Verification items for the finished model (mm, model axes). Face numbers are marked on the shaded views. Round coordinates to 2 decimals unless told otherwise and drop trailing zeros. Loops run counter-clockwise (first coordinate to the right, second up) from the corner with the lowest first, then second, coordinate; pieces in that order, holes last. Notation, with made-up numbers: M -15,-21 L 16,-21 A22 ccw 16,4 Z; hole C -18.5,3.25 d7. An arc over 180 degrees is marked long. One line per item, written item: value.
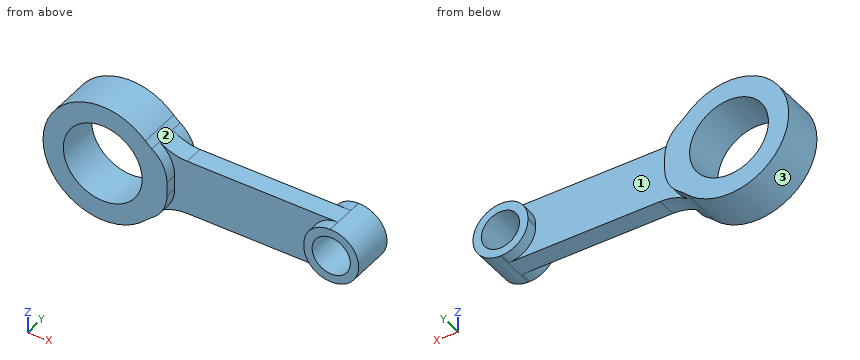
from build123d import *

# Parameters (mm, degrees)
F0_R          = 16.5
F0_R_2        = 8
F1_DEPTH      = 17.9
F2_W          = 57.2901275009
F2_H          = 11.0436469637
F2_H_2        = 10.7600754127
F3_DEPTH      = 25.001
F3_DEPTH_BACK = 25.001
F4_R          = 11
F5_R          = 11
F6_R          = 11
F7_R          = 15


with BuildPart() as f1:
    # F0 (on Front) → F1 (new body)
    with BuildSketch(Plane.XZ):
        with BuildLine():
            Line((32.137329833, -11.4990798469), (95.5545260385, -11.4990798469))
            Line((95.5545260385, -11.4990798469), (95.8454739615, -11.4990798469))
            ThreePointArc((95.8454739615, -11.4990798469), (107.1962842582, 0.2923153343), (95.2608909699, 11.4916136056))
            Line((95.2608909699, 11.4916136056), (32.1446460941, 11.4916136056))
            ThreePointArc((32.1446460941, 11.4916136056), (24.3962738222, 13.0535354211), (17.858136719, 17.495340892))
            ThreePointArc((17.858136719, 17.495340892), (-24.9999998314, 0.0029037072), (17.8540721294, -17.4994888039))
            ThreePointArc((17.8540721294, -17.4994888039), (24.3910991645, -13.0601018267), (32.137329833, -11.4990798469))
        make_face()
        Circle(F0_R, mode=Mode.SUBTRACT)
        with Locations((95.7, 0)):
            Circle(F0_R_2, mode=Mode.SUBTRACT)
    extrude(amount=F1_DEPTH)

    # F2 (on Top) → F3 (cut, two sides)
    with BuildSketch(Plane.XY) as f3_sk:
        with Locations((55.5549362496, 0.6468234818)):
            Rectangle(F2_W, F2_H)
        with Locations((55.5549362496, -18.4050377063)):
            Rectangle(F2_W, F2_H_2)
    extrude(amount=-F3_DEPTH, mode=Mode.SUBTRACT)
    extrude(f3_sk.sketch, amount=F3_DEPTH_BACK, mode=Mode.SUBTRACT)

    # F4
    f4_edges = [f1.edges().sort_by_distance(p)[0] for p in [
        (84.2, -2.4375, -11.49908),
    ]]
    fillet(f4_edges, radius=F4_R)

    # F5
    f5_edges = [f1.edges().sort_by_distance(p)[0] for p in [
        (84.2, -2.4375, 11.491614),
    ]]
    fillet(f5_edges, radius=F5_R)

    # F6
    f6_edges = [f1.edges().sort_by_distance(p)[0] for p in [
        (84.2, -15.4625, -11.49908),
        (84.2, -15.4625, 11.491614),
    ]]
    fillet(f6_edges, radius=F6_R)

    # F7
    f7_edges = [f1.edges().sort_by_distance(p)[0] for p in [
        (26.909872, -2.4375, -12.194322),
        (26.909872, -2.4375, 12.188838),
        (26.909872, -15.4625, -12.194322),
        (26.909872, -15.4625, 12.188838),
    ]]
    fillet(f7_edges, radius=F7_R)


solid = f1.part
(1) Sectioned sample at A-A on y = -8.5. Enter the section's corners in (x, z), and give its area (3 significant figures).
Completed:
outline: M 17.85,-17.5 A20 cw 32.14,-11.5 L 95.85,-11.5 A11.5 ccw long 95.26,11.49 L 32.14,11.49 A20 cw 17.86,17.5 A25 ccw long Z; hole C 0,0 d33; hole C 95.7,0 d16
area: 2,790 mm^2
(2) Mould release check, pull along X, two halves, no side actions. Record for the marked faces 1, 2 and 3: +X half, -X half, draft (parallel to the pull), parting line (faces both ways), or undercut.
Completed:
face 1: undercut
face 2: +X half
face 3: parting line
(3) Sectioned sample at D-D on x = 92. Enter the section's corners in (y, z) (3 decimals), and give its area (3 significant figures).
Completed:
outline: M -17.9,-11.023 L -13.025,-11.023 L -13.025,-11.499 L -4.875,-11.499 L -4.875,-11.023 L 0,-11.023 L 0,-7.093 L -17.9,-7.093 Z; M -17.9,7.093 L 0,7.093 L 0,11.016 L -4.875,11.016 L -4.875,11.492 L -13.025,11.492 L -13.025,11.016 L -17.9,11.016 Z
area: 148 mm^2
(4) Depth check by flat-ended pin: pin 1 Ø4 at (x, y) = (-5.5, -14.5) entering from +Z; pin 2 Ø1.5 at (y, z) = (-2, -1.5) entering from +X; pin 3 Ø1.5 at (y, z) = (-4.5, 20) entering from -X. Enter the tip coordinate at first touch or a pass-through.
Completed:
pin 1: stops at z = 24.75
pin 2: stops at x = 107.18
pin 3: stops at x = -15.95
(5) Sectioned sample at B-B on x = 0. Enter the section's corners in (y, z), and give its area (3 significant figures).
Completed:
outline: M -17.9,-25 L 0,-25 L 0,-16.5 L -17.9,-16.5 Z; M -17.9,16.5 L 0,16.5 L 0,25 L -17.9,25 Z
area: 304 mm^2
(6) Thickness scan on L1, parallel to X at y = -9.75, z = 0.5 (3 decimals); L2, parallel to X at y = -15, z = 5.5; L3, parallel to Z at x = 95.7, y = -10.5. Record the ranges inside material, lowest first. Write a range as from..to.
Completed:
L1: x = -24.995..-16.492, 16.492..87.716, 103.684..107.189
L2: x = -24.39..-15.56, 15.56..26.69, 85.41..89.89, 101.51..105.8
L3: z = -11.5..-8, 8..11.5
(7) Sectioned sample at C-C on z = -5.5. Enter the section's corners in (x, y) (1 decimal), and give its area (3 significant figures).
Completed:
outline: M -24.4,-17.9 L -15.6,-17.9 L -15.6,0 L -24.4,0 Z; M 15.6,-17.9 L 26.7,-17.9 L 26.7,-13 L 85.4,-13 L 85.4,-17.9 L 89.9,-17.9 L 89.9,0 L 85.4,0 L 85.4,-4.9 L 26.7,-4.9 L 26.7,0 L 15.6,0 Z; M 101.5,-17.9 L 105.8,-17.9 L 105.8,0 L 101.5,0 Z
area: 993 mm^2
